from build123d import *

# Parameters (mm, degrees)
SKETCH1_W           = 140
SKETCH1_H           = 80
BOSS_EXTRUDE1_DEPTH = 25
SKETCH2_W           = 30
SKETCH2_H           = 60
BOSS_EXTRUDE2_DEPTH = 110
FILLET1_R           = 70
BOSS_EXTRUDE4_DEPTH = 30
SKETCH6_W           = 105
SKETCH6_H           = 80
BOSS_EXTRUDE5_DEPTH = 20
CUT_EXTRUDE1_DEPTH  = 188.949461292
CHAMFER1_SIZE       = 15
CHAMFER1_SIZE2      = 4.019237886
BOSS_EXTRUDE8_DEPTH = 25
SKETCH14_W          = 40
SKETCH14_H          = 15
CUT_EXTRUDE4_DEPTH  = 20
FILLET2_R           = 15


with BuildPart() as part:
    # Sketch1 → Boss-Extrude1 (new body)
    with BuildSketch(Plane(origin=(0, 0, 0), x_dir=(1, 0, 0), z_dir=(0, 1, 0))):
        Rectangle(SKETCH1_W, SKETCH1_H)
    extrude(amount=BOSS_EXTRUDE1_DEPTH)

    # Sketch2 → Boss-Extrude2 (add)
    with BuildSketch(Plane(origin=(0, 25, 0), x_dir=(1, 0, 0), z_dir=(0, 1, 0))):
        with Locations((45, -1.000466796)):
            Rectangle(SKETCH2_W, SKETCH2_H)
    extrude(amount=BOSS_EXTRUDE2_DEPTH)

    # Fillet1
    fillet1_edges = [part.edges().sort_by_distance(p)[0] for p in [
        (30, 25, 1.000466796),
    ]]
    fillet(fillet1_edges, radius=FILLET1_R)

    # Sketch4 → Boss-Extrude4 (add)
    with BuildSketch(Plane(origin=(0, 25, 0), x_dir=(1, 0, 0), z_dir=(0, 1, 0))):
        with BuildLine():
            ThreePointArc((-40, 14.142135624), (-53.660254038, 12.247448714), (-60, 0))
            Line((-60, 0), (-55, 0))
            ThreePointArc((-55, 0), (-50, 8.660254038), (-40, 8.660254038))
            Line((-40, 8.660254038), (-40, 14.142135624))
        make_face()
        with BuildLine():
            Line((-55, 0), (-60, 0))
            ThreePointArc((-60, 0), (-53.660254038, -12.247448714), (-40, -14.142135624))
            Line((-40, -14.142135624), (-40, -8.660254038))
            ThreePointArc((-40, -8.660254038), (-50, -8.660254038), (-55, 0))
        make_face()
        with BuildLine():
            ThreePointArc((-30, 0), (-32.752551286, 8.660254038), (-40, 14.142135624))
            Line((-40, 14.142135624), (-40, 8.660254038))
            ThreePointArc((-40, 8.660254038), (-36.339745962, 5), (-35, 0))
            ThreePointArc((-35, 0), (-36.339745962, -5), (-40, -8.660254038))
            Line((-40, -8.660254038), (-40, -14.142135624))
            ThreePointArc((-40, -14.142135624), (-32.752551286, -8.660254038), (-30, 0))
        make_face()
    extrude(amount=BOSS_EXTRUDE4_DEPTH)

    # Sketch6 → Boss-Extrude5 (add)
    with BuildSketch(Plane(origin=(0, 135, 0), x_dir=(1, 0, 0), z_dir=(0, 1, 0))):
        with Locations((17.5, 0)):
            Rectangle(SKETCH6_W, SKETCH6_H)
    extrude(amount=BOSS_EXTRUDE5_DEPTH)

    # Sketch7 → Cut-Extrude1 (cut, through all)
    with BuildSketch(Plane.XY.offset(40)):
        with BuildLine():
            ThreePointArc((48, 155), (38, 165), (28, 155))
            Line((28, 155), (38, 155))
            Line((38, 155), (48, 155))
        make_face()
        with BuildLine():
            Line((38, 155), (28, 155))
            ThreePointArc((28, 155), (38, 145), (48, 155))
            Line((48, 155), (38, 155))
        make_face()
    extrude(amount=-CUT_EXTRUDE1_DEPTH, mode=Mode.SUBTRACT)

    # Chamfer1
    chamfer1_edges = [part.edges().sort_by_distance(p)[0] for p in [
        (70, 155, 0),
    ]]
    chamfer1_side = [part.faces().sort_by_distance(p)[0] for p in [
        (59, 155, 0),
    ]]
    chamfer(chamfer1_edges, length=CHAMFER1_SIZE, length2=CHAMFER1_SIZE2, reference=chamfer1_side[0])

    # Sketch13 → Boss-Extrude8 (add)
    with BuildSketch(Plane(origin=(0, 25, 0), x_dir=(1, 0, 0), z_dir=(0, 1, 0))):
        with BuildLine():
            Line((-40, -14.142135624), (-40, -15))
            Line((-40, -15), (16, -15))
            Line((16, -15), (16, 15))
            Line((16, 15), (-40, 15))
            Line((-40, 15), (-40, 14.142135624))
            ThreePointArc((-40, 14.142135624), (-32.752551286, 8.660254038), (-30, 0))
            ThreePointArc((-30, 0), (-32.752551286, -8.660254038), (-40, -14.142135624))
        make_face()
    extrude(amount=BOSS_EXTRUDE8_DEPTH)

    # Sketch14 → Cut-Extrude4 (cut)
    with BuildSketch(Plane(origin=(0, 155, 0), x_dir=(1, 0, 0), z_dir=(0, 1, 0))):
        with Locations((-15, 32.5)):
            Rectangle(SKETCH14_W, SKETCH14_H)
        with Locations((-15, -32.5)):
            Rectangle(SKETCH14_W, SKETCH14_H)
    extrude(amount=-CUT_EXTRUDE4_DEPTH, mode=Mode.SUBTRACT)

    # Fillet2
    fillet2_edges = [part.edges().sort_by_distance(p)[0] for p in [
        (5, 145, -25),
        (5, 145, 25),
    ]]
    fillet(fillet2_edges, radius=FILLET2_R - 0.0001)  # a hair under: the kernel refuses the full size


solid = part.part
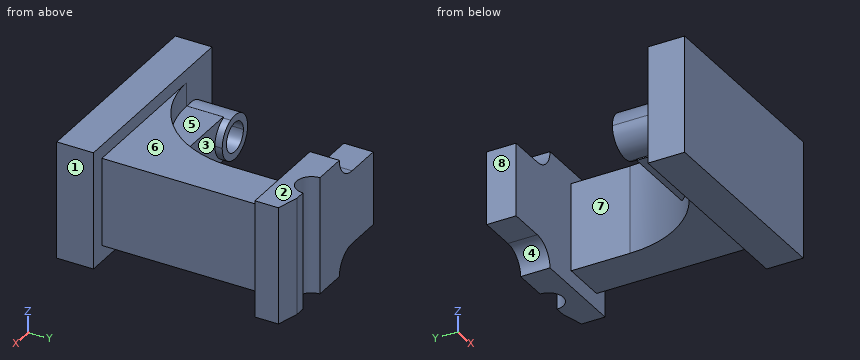
Here's how the part is built. I have some questions about the finished solid (model axes, mm). Face numbers are marked on the shaded views. A direction names the side the tool comes from. Coordinates: 2 decimals unless noted, no trailing zeros. Loops run counter-clockwise (first coordinate to the right, second up) from the corner with the lowest first, then second, coordinate; pieces in that order, holes last. Notation, with made-up numbers: (-13.5, 22.25) -> (19.5, 22.25) arc R15 ccw to (19.5, 32.25) -> close; hole circle Ø5 at (83.25, 56.5). An arc over 180 degrees is marked (long way). Use one line per item in the form item = value. Start each with the question number.
(1) We'd pull the mould along X, two halves only. Please class the marked faces 1, 2 and 3: pulls with the +X half, pulls with the -X half, needs draft (parallel to the pull), parting line crosses it, or undercut.
(2) Please list where these lines run through material, in increasing order: line 1 along Y through (x, z) = (-23, -2); line 2 along Y through (x, z) = (20, -32.5); line 3 along Z through (x, y) = (-30.5, 46).
(3) Will these pins go through, and if not, where does the flat tip stop? pin 1 (4 mm diameter, centred on y = 97.5, z = -14, fed in from -X); pin 2 (2 mm diameter, centred on y = 76, z = -4, fed in from -X); pin 3 (16 mm diameter, centred on y = 146.5, z = -7, fed in from -X); pin 4 (24 mm diameter, centred on x = -39, z = 2.5, fed in from +Y).
(4) On a 3-axis mill with a long thin cutter (end or side, diameter ignored), from which of +Z, -Z, +X, -X, +Y, -Y can I reach the whole of each face in a straight line? I mean the marked faces 4, 5, 6, 7 and 8. Say none if no direction works.
(5) If we section it at D-D (z = 29): Please give me the cut outline in (x, y), then the cut area to 3 significant figures.
(6) If we section it at C-C (y = 98): Please give me the cut outline in (x, z).
(7) If we section it at B-B (x = 52.5): Please give me the cut outline in (y, z).
(8) If we section it at A-A (x = -16): Please give me the cut outline in (y, z), then the cut area to 3 significant figures.
Verdict:
q1.face_1 = pulls with the +X half
q1.face_2 = needs draft
q1.face_3 = undercut
q2.line_1 = 0 to 50, 135 to 155
q2.line_2 = 0 to 25, 135 to 155
q2.line_3 = -15 to 15
q3.pin_1 = 30
q3.pin_2 = 27.08
q3.pin_3 = -35
q3.pin_4 = 155
q4.face_4 = -Z, -X, +Y
q4.face_5 = +Z, -X
q4.face_6 = +Z, +X, -X
q4.face_7 = +Z, -Z, -X
q4.face_8 = +Z, -Z, -X, +Y
q5.outline = (-70, 0) -> (70, 0) -> (70, 25) -> (60, 25) -> (60, 135) -> (70, 135) -> (70, 150.98) -> (55, 155) -> (48, 155) arc R10 cw to (28, 155) -> (0.2, 155) -> (0.2, 135) -> (30, 135) -> (30, 95) arc R70 cw to (-40, 25) -> (-70, 25) -> close
q5.area = 9,060 mm²
q6.outline = (30, -29) -> (60, -29) -> (60, 31) -> (30, 31) -> close
q7.outline = (0, -40) -> (25, -40) -> (25, -29) -> (135, -29) -> (135, -40) -> (155, -40) -> (155, 40) -> (135, 40) -> (135, 31) -> (25, 31) -> (25, 40) -> (0, 40) -> close
q8.outline = (0, -40) -> (25, -40) -> (25, -29) -> (29.24, -29) -> (29.24, -15) -> (50, -15) -> (50, 15) -> (29.24, 15) -> (29.24, 31) -> (25, 31) -> (25, 40) -> (0, 40) -> close; (135, -25) -> (155, -25) -> (155, 25) -> (135, 25) -> close
q8.area = 3,880 mm²
